from build123d import *

# Parameters (mm, degrees)
EXTRUDE_1_DEPTH     = 16
SKETCH_2_R          = 4.25
CUT_EXTRUDE_1_DEPTH = 5
SKETCH_3_R          = 4.25
CUT_EXTRUDE_2_DEPTH = 5
FILLET_1_R          = 4
FILLET_2_R          = 1


with BuildPart() as part:
    # Эскиз1 → Бобышка-Вытянуть1 (new body, symmetric)
    with BuildSketch(Plane.XY):
        Polygon((0, 0), (42.426406871, 42.426406871), (45.961940777, 38.890872965), (20.266663343, 13.195595531), (23.661390163, 5), (60, 5), (60, 0), align=None)
        Polygon((17.142135624, 12.899494937), (21.242640687, 3), (7.242640687, 3), align=None, mode=Mode.SUBTRACT)
    extrude(amount=EXTRUDE_1_DEPTH, both=True)

    # Эскиз2 → Вырез-Вытянуть1 (cut)
    with BuildSketch(Plane(origin=(0, 0, 0), x_dir=(0, 0, 1), z_dir=(-0.707106781, 0.707106781, 0))):
        with Locations(Location((0, 45, 0), (0, 0, 270))):  # turned: the seam where the file's is
            Circle(SKETCH_2_R)
    extrude(amount=-CUT_EXTRUDE_1_DEPTH, mode=Mode.SUBTRACT)

    # Эскиз3 → Вырез-Вытянуть2 (cut)
    with BuildSketch(Plane.XZ):
        with Locations(Location((45, 0, 0), (0, 0, 270))):  # turned: the seam where the file's is
            Circle(SKETCH_3_R)
    extrude(amount=-CUT_EXTRUDE_2_DEPTH, mode=Mode.SUBTRACT)

    # Скругление1
    fillet_1_edges = [part.edges().sort_by_distance(p)[0] for p in [
        (45.961940777, 38.890872965, 0),
        (60, 5, 0),
    ]]
    fillet(fillet_1_edges, radius=FILLET_1_R)

    # Скругление2
    fillet_2_edges = [part.edges().sort_by_distance(p)[0] for p in [
        (17.142135624, 12.899494937, 0),
        (7.242640687, 3, 0),
        (21.242640687, 3, 0),
    ]]
    fillet(fillet_2_edges, radius=FILLET_2_R)


solid = part.part
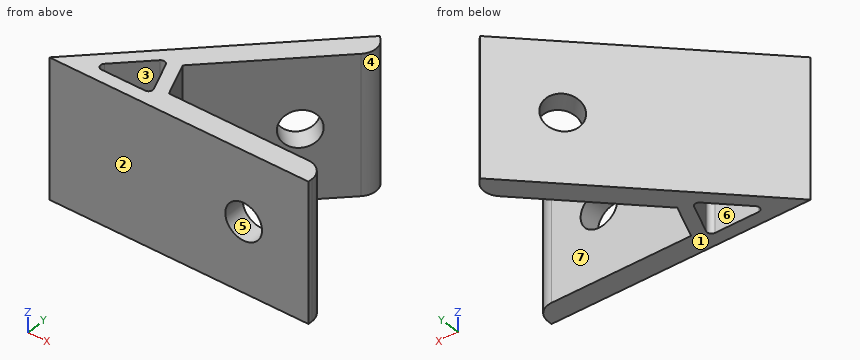
Read the model definition and answer for the solid it produces. Units are mm, in the model's axes. Face numbers are marked on the shaded views. A direction names the side the tool comes from. Coordinates: 2 decimals unless noted, no trailing zeros. Write each loop counter-clockwise with the first axis right and the second up, starting at its lowest first coordinate (ties: lowest second). Pieces come first, ordered by that corner, then holes. Notation, with made-up numbers: (8.5, 87.5) -> (52.5, 87.5) arc R33 ccw to (52.5, 124.5) -> close; hole circle Ø3 at (65.25, 56). An arc over 180 degrees is marked (long way). Return JSON: item names as keys, results as strings.
(1) Which of the six approach directions +Z, -Z, +X, -X, +Y, -Y give full straight-line access (tool end or side, diameter ignored) to the marked faces 5, 6 and 7?
Answers below:
{"face 5": "-Y", "face 6": "+Z, -Z", "face 7": "+Z, -Z, +X"}
(2) The part is cut by section D-D on x = 28. Give the vertices of the cut face in (y, z).
Answers below:
{"outline": "(0, -16) -> (5, -16) -> (5, 16) -> (0, 16) -> close; (20.93, -16) -> (28, -16) -> (28, 16) -> (20.93, 16) -> close"}
(3) The part is cut by section C-C on z = -11. Give the vertices of the cut face in (x, y).
Answers below:
{"outline": "(0, 0) -> (60, 0) -> (60, 1) arc R4 ccw to (56, 5) -> (23.66, 5) -> (20.27, 13.2) -> (43.13, 36.06) arc R4 ccw to (43.13, 41.72) -> (42.43, 42.43) -> close; hole (8.95, 4.71) arc R1 ccw to (9.66, 3) -> (19.75, 3) arc R1 ccw to (20.67, 4.38) -> (17.71, 11.52) arc R1 ccw to (16.08, 11.84) -> close"}
(4) For a pull along Y with two mould halves and no side action, classify the marked faces 1, 2, 3 and 4 as pulls with the +Y half, pulls with the -Y half, needs draft (parallel to the pull), parting line crosses it, or undercut.
Answers below:
{"face 1": "needs draft", "face 2": "pulls with the -Y half", "face 3": "undercut", "face 4": "undercut"}
(5) The part is cut by section B-B on x = 45. Give the vertices of the cut face in (y, z).
Answers below:
{"outline": "(0, -16) -> (5, -16) -> (5, -4.25) -> (0, -4.25) -> close; (0, 4.25) -> (5, 4.25) -> (5, 16) -> (0, 16) -> close"}
(6) Each of these flat-tipped pins is pushed along its axis until it touches: P1, Ø2, axis at x = 21, z = -7, coming from the +Y side; P2, Ø5, axis at y = 7.5, z = 8.5, coming from the -X side; P3, Ø5, axis at y = 13, z = -1, coming from the +X side; P4, Ø5, axis at x = 25.5, y = 31.5, coming from the +Z side. Where does it stop, or does it pass through?
Answers below:
{"P1": "y = 22", "P2": "x = 5", "P3": "x = 22.57", "P4": "through"}
(7) The part is cut by section A-A on z = -2.5. Give the vertices of the cut face in (x, y), then the cut area to 3 significant figures.
Answers below:
{"outline": "(0, 0) -> (41.56, 0) -> (41.56, 5) -> (23.66, 5) -> (20.27, 13.2) -> (32.93, 25.85) -> (29.39, 29.39) -> close; (34.25, 34.25) -> (37.79, 30.71) -> (43.13, 36.06) arc R4 ccw to (43.13, 41.72) -> (42.43, 42.43) -> close; (48.44, 0) -> (60, 0) -> (60, 1) arc R4 ccw to (56, 5) -> (48.44, 5) -> close; hole (8.95, 4.71) arc R1 ccw to (9.66, 3) -> (19.75, 3) arc R1 ccw to (20.67, 4.38) -> (17.71, 11.52) arc R1 ccw to (16.08, 11.84) -> close", "area": "445 mm^2"}
(8) Consider line 1 along X through (y, z) = (4, 0); line 2 along Y through (x, z) = (27.5, 14.5); line 3 along Y through (x, z) = (13, 0.5). Determine where each line is inside the solid, lowest interval first. Write a range as from..to.
Answers below:
{"line 1": "4..8.66, 20.75..40.75, 49.25..58.65", "line 2": "0..5, 20.43..27.5", "line 3": "0..3, 8.76..13"}
